from build123d import *

# Parameters (mm, degrees)
F1_DEPTH      = 3
F1_DEPTH_BACK = 3
F0_R          = 11.25
F2_DEPTH      = 3
F3_DEPTH      = 3


with BuildPart() as f1:
    # F0 (on Right) → F1 (new body, two sides)
    with BuildSketch(Plane.YZ) as f1_sk:
        with BuildLine():
            ThreePointArc((0, 22.5), (15.909903, 15.909903), (22.5, 0))
            ThreePointArc((22.5, 0), (15.909903, -15.909903), (0, -22.5))
            Line((0, -22.5), (55, -22.5))
            ThreePointArc((55, -22.5), (32.5, 0), (55, 22.5))
            Line((55, 22.5), (0, 22.5))
        make_face()
    extrude(amount=F1_DEPTH)
    extrude(f1_sk.sketch, amount=-F1_DEPTH_BACK)

    # F0 (on Right) → F2 (join)
    with BuildSketch(Plane.YZ):
        with BuildLine():
            ThreePointArc((0, -22.5), (15.909903, -15.909903), (22.5, 0))
            ThreePointArc((22.5, 0), (15.909903, 15.909903), (0, 22.5))
            ThreePointArc((0, 22.5), (-22.5, 0), (0, -22.5))
        make_face()
        Circle(F0_R, mode=Mode.SUBTRACT)
    extrude(amount=F2_DEPTH)

    # F0 (on Right) → F3 (join)
    with BuildSketch(Plane.YZ):
        with BuildLine():
            ThreePointArc((77.5, 0), (70.909903, 15.909903), (55, 22.5))
            ThreePointArc((55, 22.5), (32.5, 0), (55, -22.5))
            ThreePointArc((55, -22.5), (70.909903, -15.909903), (77.5, 0))
        make_face()
        with Locations((55, 0)):
            Circle(F0_R, mode=Mode.SUBTRACT)
    extrude(amount=-F3_DEPTH)


solid = f1.part
Here's how the part is built. I have some questions about the finished solid (model axes, mm). A direction names the side the tool comes from. Coordinates: 2 decimals unless noted, no trailing zeros. Loops run counter-clockwise (first coordinate to the right, second up) from the corner with the lowest first, then second, coordinate; pieces in that order, holes last. Notation, with made-up numbers: (33, -26.5) -> (68, -26.5) arc R6 ccw to (68, -21.5) -> close; hole circle Ø8 at (85.5, 40.25). An arc over 180 degrees is marked (long way). Use one line per item in the form item = value. Start each with the question number.
(1) If we section it at D-D (z = 9): Please give me the cut outline in (x, y).
(2) If we section it at C-C (y = 63): Please give me the cut outline in (x, z), then the cut area to 3 significant figures.
(3) If we section it at B-B (z = -6): Please give me the cut outline in (x, y), then the cut area to 3 significant figures.
(4) We'd pull the mould along Z, two halves only. Please class faces 1 (the face through (3, 16, 0)), 2 (the face through (1.521, 32.505, -0.495)), 3 (the face through (0, 27, -22.5)): pulls with the +Z half, pulls with the -Z half, needs draft (parallel to the pull), parting line crosses it, or undercut.
(5) If we section it at A-A (x = 0.95): Please give me the cut outline in (y, z), then the cut area to 3 significant figures.
(6) Please list where these lines run through material, in increasing order: line 1 along Z through (x, y) = (-2.4, 55); line 2 along X through (y, z) = (72, 5); line 3 along X through (y, z) = (17, 7.5).
(7) On a 3-axis mill with a long thin cutter (end or side, diameter ignored), from which of +Z, -Z, +X, -X, +Y, -Y can I reach the whole of each face in a straight line? I mean faces 4 (the face through (0, 44.7, 5.3)), 5 (the face through (0, -10.3, 5.3)), 6 (the face through (1.479, -22.495, 0.495)). Say none if no direction works.
(8) Will this pin go through, and if not, where does the flat tip stop? pin 1 (13.5 mm diameter, centred on y = 48, z = -10, fed in from +X).
Verdict:
q1.outline = (-3, 20.62) -> (0, 20.62) -> (0, 6.75) -> (3, 6.75) -> (3, 34.38) -> (0, 34.38) -> (0, 48.25) -> (-3, 48.25) -> close; (-3, 61.75) -> (0, 61.75) -> (0, 75.62) -> (-3, 75.62) -> close; (0, -20.62) -> (3, -20.62) -> (3, -6.75) -> (0, -6.75) -> close
q2.outline = (-3, -21.03) -> (0, -21.03) -> (0, -7.91) -> (-3, -7.91) -> close; (-3, 7.91) -> (0, 7.91) -> (0, 21.03) -> (-3, 21.03) -> close
q2.area = 78.7 mm²
q3.outline = (-3, 21.69) -> (0, 21.69) -> (0, 9.52) -> (3, 9.52) -> (3, 33.31) -> (0, 33.31) -> (0, 45.48) -> (-3, 45.48) -> close; (-3, 64.52) -> (0, 64.52) -> (0, 76.69) -> (-3, 76.69) -> close; (0, -21.69) -> (3, -21.69) -> (3, -9.52) -> (0, -9.52) -> close
q3.area = 216 mm²
q4.face_1 = needs draft
q4.face_2 = undercut
q4.face_3 = pulls with the -Z half
q5.outline = (0, -22.5) -> (55, -22.5) arc R22.5 cw to (55, 22.5) -> (0, 22.5) arc R22.5 ccw to start; hole circle Ø22.5 at (0, 0)
q5.area = 2,080 mm²
q6.line_1 = -22.5 to -11.25, 11.25 to 22.5
q6.line_2 = -3 to 0
q6.line_3 = 0 to 3
q7.face_4 = +X, +Y
q7.face_5 = -X, -Y
q7.face_6 = +X, -X, -Y
q8.pin_1 = 0
